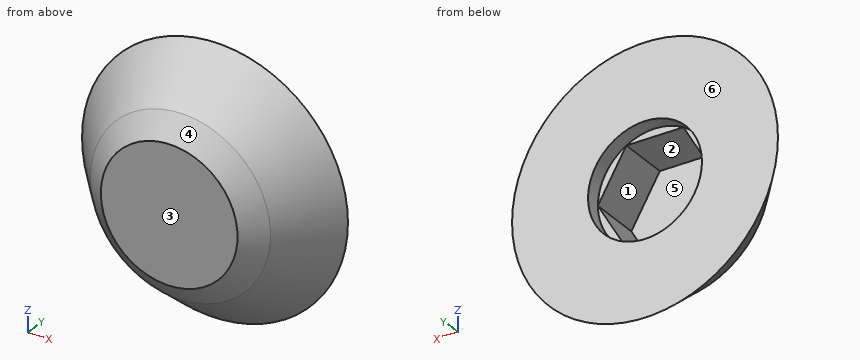
```python
from build123d import *

# Parameters (mm, degrees)
SCHIZZO4_R               = 7.5
TAGLIO_ESTRUSIONE1_DEPTH = 2
TAGLIO_ESTRUSIONE2_DEPTH = 6.8


with BuildPart() as part:
    # Schizzo3 → Rivoluzione1 (revolve)
    with BuildSketch(Plane.XY):
        Polygon((-17.5, 9.3), (0, 9.3), (0, 0), (-9, 0), (-11.850227939, 2.294282645), align=None)
    revolve(axis=Axis((0, 9.3, 0), (0, -1, 0)))

    # Schizzo4 → Taglio-Estrusione1 (cut)
    with BuildSketch(Plane(origin=(0, 9.3, 0), x_dir=(1, 0, 0), z_dir=(0, 1, 0))):
        with Locations(Location((0, 0, 0), (0, 0, 270))):
            Circle(SCHIZZO4_R)
    extrude(amount=-TAGLIO_ESTRUSIONE1_DEPTH, mode=Mode.SUBTRACT)

    # Schizzo5 → Taglio-Estrusione2 (cut)
    with BuildSketch(Plane(origin=(0, 7.3, 0), x_dir=(1, 0, 0), z_dir=(0, 1, 0))):
        Polygon((3.75277675, -6.5), (7.505553499, 0), (3.75277675, 6.5), (-3.75277675, 6.5), (-7.505553499, 0), (-3.75277675, -6.5), align=None)
    extrude(amount=-TAGLIO_ESTRUSIONE2_DEPTH, mode=Mode.SUBTRACT)


solid = part.part
```
Source: CAD feature listing. Evaluate the final solid. Frame: model axes, mm. Face numbers are marked on the shaded views. A direction names the side the tool comes from. Give positions to 0.01 mm unless a question says otherwise; leave off trailing zeros. Write each loop counter-clockwise with the first axis right and the second up, starting at its lowest first coordinate (ties: lowest second). Pieces come first, ordered by that corner, then holes.
1. Access query for the marked faces 5 and 6. Directions: +Z, -Z, +X, -X, +Y, -Y. A direction counts if a zero-diameter tool reaches every point of the face in a straight line with its end or side. Return the directions, or none.
2. Pull-direction query (Z, two-part tool) for the marked faces 1, 2, 3 and 4; classes: +Z half, -Z half, draft (parallel to the pull), parting line (faces both ways), or undercut.
3. Material intervals for line 1 along Y through (x, z) = (4, 2); line 2 along Y through (x, z) = (-6.5, 2); line 3 along Z through (x, y) = (0, 8.4), sorted ascending.
4. Section query C-C (y = 8.75). Return the cut outline in (x, z), then the cut area to 3 significant figures.
5. Section query A-A (x = 0). Return the cut outline in (y, z).
6. First-contact query: pin 1 (12 mm diameter, centred on x = -8.5, z = 11.5, fed in from -Y); pin 2 (4 mm diameter, centred on x = 5, z = -1.5, fed in from +Y); pin 3 (6 mm diameter, centred on x = -8, z = -11, fed in from -Y); pin 4 (2 mm diameter, centred on y = 7, z = 12, fed in from +X). Flat tips, straight axial feed; report the tip coordinate or a pass-through.
7. Section query B-B (y = 5.5). Return the cut outline in (x, z).
Output values:
1. face 5: +Y
1. face 6: +Z, -Z, +X, -X, +Y
2. face 1: undercut
2. face 2: undercut
2. face 3: draft
2. face 4: parting line
3. line 1: y = 0 to 0.5
3. line 2: y = 0 to 7.3
3. line 3: z = -16.77 to -7.5, 7.5 to 16.77
4. outline: circle Ø34.11 at (0, 0); hole circle Ø15 at (0, 0)
4. area: 737 mm2
5. outline: (0, -9) - (2.29, -11.85) - (9.3, -17.5) - (9.3, -7.5) - (7.3, -7.5) - (7.3, -6.5) - (0.5, -6.5) - (0.5, 6.5) - (7.3, 6.5) - (7.3, 7.5) - (9.3, 7.5) - (9.3, 17.5) - (2.29, 11.85) - (0, 9) - close
6. pin 1: stops at y = 0
6. pin 2: stops at y = 7.3
6. pin 3: stops at y = 1.29
6. pin 4: stops at x = 11.64
7. outline: circle Ø28.87 at (0, 0); hole (-7.51, 0) - (-3.75, -6.5) - (3.75, -6.5) - (7.51, 0) - (3.75, 6.5) - (-3.75, 6.5) - close
